Can you work these out from the model? Positions are in its coordinate system, mm. Face numbers are marked on the shaded views. A direction names the side the tool comes from. Give positions to 0.01 mm unless a question says otherwise; leave off trailing zeros. Order: outer loops, then holes, each group sorted by start corner. A loop starts at its lowest first (then second) coordinate and runs counter-clockwise, first axis right, second up. Notation, with made-up numbers: (-4, 70.5) - (49, 70.5) arc R21 cw to (49, 96.5) - close; hole circle Ø8 at (56.5, 65.5). An arc over 180 degrees is marked (long way). Use one line per item in the form item = value. Start each with the question number.
1) Which directions (+Z, -Z, +X, -X, +Y, -Y) give clear straight access to the entire face, cutting with the end or side of a thin tool? Please do the marked faces 1 and 2.
2) Suppose I cut it at C-C, the plane x = 26.5. Write out the boundary of the cut face in (y, z).
3) Suppose I cut it at B-B, the plane y = 5. State how many separate pieces and enclosed holes the cut face has, and give its area (3 significant figures).
4) Please list where these lines run through material, in increasing order: probe 1 along X at (y, z) = (2.25, 6); probe 2 along Z at (x, y) = (29, 4); probe 3 along Z at (x, y) = (33.5, 0.5).
5) Suppose I cut it at A-A, the plane z = 3. Write out the boundary of the cut face in (x, y), and give its area (3 significant figures).
6) Suppose I cut it at D-D, the plane y = 1.5. Write out the boundary of the cut face in (x, z).
7) We'd pull the mould along Z, two halves only. Please class the marked faces 3, 4 and 5: released by +Z, released by -Z, zero draft, split by the parting line, or undercut.
8) For pin 1 (0.6 mm diameter, centred on x = 33.5, y = 4.5, fed in from +Z); pin 2 (2 mm diameter, centred on x = 33, y = 4, fed in from -Z); pin 3 (12 mm diameter, centred on x = 3.5, z = 1.5, fed in from +Y); pin 4 (1.6 mm diameter, centred on x = 17.5, z = 10.5, fed in from -Y), each with a flat end and sliding along its axis, tell me the tip position at first contact or that it passes through.
Autodesk Inventor part; units mm, degrees
ref_plane "YZ Plane" through (0, 0, 0) normal (1, 0, 0) x (0, 1, 0)
ref_plane "XZ Plane" through (0, 0, 0) normal (0, 1, 0) x (-1, 0, 0)
ref_plane "XY Plane" through (0, 0, 0) normal (0, 0, 1) x (1, 0, 0)
sketch "Sketch1" plane through (0, 0, 0) normal (0, 1, 0) x (-1, 0, 0)
  line L0 (-0.5, 11) -> (0.5, 11) construction
  line L1 (0.5, 11) -> (0.5, -11) construction
  line L2 (0.5, -11) -> (-0.5, -11) construction
  line L3 (-0.5, -11) -> (-0.5, 11) construction
  line L4 (-0.5, 11) -> (0.5, -11) construction
  line L5 (0.5, 11) -> (-0.5, -11) construction
  line L6 (-0.5, 11) -> (-0.5, 9.9373) construction
  line L7 (-1.5, 10) -> (-1.5, 12)
  line L8 (-1.5, 12) -> (1.5, 12)
  line L9 (1.5, 12) -> (1.5, 10)
  line L10 (1.5, 10) -> (-1.5, 12) construction
  line L11 (-1.5, 10) -> (1.5, 12) construction
  line L12 (-0.5, 11) -> (0.5, 11)
  line L13 (0.5, 11) -> (0.5, 10)
  line L14 (-0.5, 10) -> (-0.5, 11)
  line L15 (1.5, 10) -> (0.5, 10)
  line L16 (-0.5, 10) -> (-1.5, 10)
  line L17 (-34.5, 0) -> (-32.5, 0)
  line L18 (-32.5, 0) -> (-32.5, 10)
  line L19 (-32.5, 10) -> (-34.5, 10)
  line L20 (-34.5, 10) -> (-34.5, 0)
  line L21 (-32.5, 10) -> (-1.5, 12)
  line L22 (-1.5, 10) -> (-32.5, 8)
  point P0 (0, 0)
  point P1 (0, 11)
  dimension "d0" = 1
  dimension "d1" = 22
  dimension "d2" = 3
  dimension "d3" = 2
  dimension "d4" = 2
  dimension "d5" = 10
  dimension "d6" = 35
extrude "Extrusion1" add sketch "Sketch1" along normal blind 10
mirror "Mirror1" about plane through (34.5, 0, 0) normal (0, 0, -1) of "Extrusion1"
draft "FaceDraft1" angle 6 pull direction (-1, 0, 0) faces at (11.8333, 10, -10.6667) fixed edges at (34.5, 10, 0)
sketch "Sketch2" plane through (1.5, 0, -12) normal (0, 0, -1) x (-1, 0, 0)
  line L0 (-15, 5.5) -> (-17, 5.5)
  line L1 (-17, 5.5) -> (-17, 2.5)
  line L2 (-17, 2.5) -> (-15, 2.5)
  line L3 (-15, 2.5) -> (-15, 5.5)
  line L4 (-15, 5.5) -> (-17, 2.5) construction
  line L5 (-17, 5.5) -> (-15, 2.5) construction
  line L6 (0, 0) -> (-31, 0)
  line L7 (3, 0) -> (3, 6.2162)
  point P0 (1.5, 0)
  point P1 (-16, 4)
  dimension "d10" = 2
  dimension "d11" = 3
  dimension "d12" = 2.5
  dimension "d13" = 18
extrude "Extrusion2" cut sketch "Sketch2" against normal through all
sketch "Sketch3" plane through (32.5, 0, -8) normal (-1, 0, 0) x (0, 0, 1)
  line L0 (13, 5) -> (3, 5) construction
  line L1 (13, 6.25) -> (3, 6.25)
  line L2 (3, 3.75) -> (13, 3.75)
  arc A0 (13, 3.75) -> (13, 6.25) centre (13, 5) ccw
  arc A1 (3, 6.25) -> (3, 3.75) centre (3, 5) ccw
  point P0 (8, 0)
  point P1 (8, 5)
  dimension "d16" = 5
  dimension "d17" = 2.5
extrude "Extrusion3" cut sketch "Sketch3" against normal through all
move faces "Move1" translate (-0.5, 0, 0) faces at (-1.5, 4.1442, -11.3333) (-1.5, 4.1442, 11.3333)
properties part number "holder"
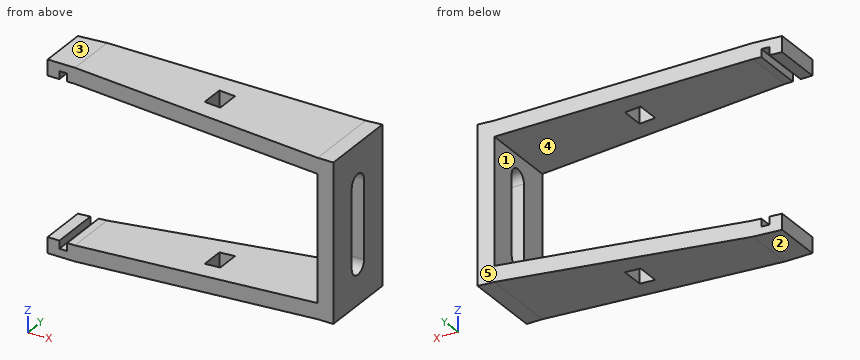
Result sheet:
q1.face_1 = -X, +Y, -Y
q1.face_2 = -Z, +X, -X, +Y, -Y
q2.outline = (0, -10.39) - (9.16, -10.39) - (9.16, -8.39) - (0, -8.39) - close; (0, 8.39) - (9.16, 8.39) - (9.16, 10.39) - (0, 10.39) - close
q3.separate_pieces = 4
q3.enclosed_holes = 0
q3.area = 143 mm²
q4.probe_1 = 32.5 to 34.5
q4.probe_2 = -10.23 to -8.23, 8.23 to 10.23
q4.probe_3 = -10 to 10
q5.outline = (32.5, 0) - (34.5, 0) - (34.5, 3.75) - (32.5, 3.75) - close; (32.5, 6.25) - (34.5, 6.25) - (34.5, 10) - (32.5, 9.79) - close
q5.area = 14.8 mm²
q6.outline = (-2, -12) - (1.5, -12) - (32.5, -10) - (34.5, -10) - (34.5, 10) - (32.5, 10) - (1.5, 12) - (-2, 12) - (-2, 10) - (-0.5, 10) - (-0.5, 11) - (0.5, 11) - (0.5, 10) - (1.5, 10) - (32.5, 8) - (32.5, -8) - (1.5, -10) - (0.5, -10) - (0.5, -11) - (-0.5, -11) - (-0.5, -10) - (-2, -10) - close
q7.face_3 = released by +Z
q7.face_4 = undercut
q7.face_5 = zero draft
q8.pin_1 = 10
q8.pin_2 = -10.03
q8.pin_3 = through
q8.pin_4 = 0
